from build123d import *

# Parameters (mm, degrees)
SKETCH1_W           = 254
SKETCH1_H           = 127
BOSS_EXTRUDE1_DEPTH = 6.35
SKETCH4_W           = 52.216720723
SKETCH4_H           = 76.2
SKETCH4_R           = 8.89
SKETCH4_R_2         = 12.7
SKETCH4_R_3         = 7.62
SKETCH4_R_4         = 3.175
CUT_EXTRUDE3_DEPTH  = 285.051619429


with BuildPart() as part:
    # Sketch1 → Boss-Extrude1 (new body)
    with BuildSketch(Plane.XY):
        with Locations((127, 63.5)):
            Rectangle(SKETCH1_W, SKETCH1_H)
    extrude(amount=BOSS_EXTRUDE1_DEPTH)

    # Sketch4 → Cut-Extrude3 (cut, through all)
    # profile 1 of 8: a face of its own
    with BuildSketch(Plane.XY.offset(6.35)):
        with Locations((69.998360362, 70.4)):
            Rectangle(SKETCH4_W, SKETCH4_H)
        with Locations((69.925, 95.8)):
            Circle(SKETCH4_R, mode=Mode.SUBTRACT)
        with Locations((69.925, 58.97)):
            Circle(SKETCH4_R_2, mode=Mode.SUBTRACT)
    # profile 2 of 8: a face of its own
    with BuildSketch(Plane.XY.offset(6.35)):
        with Locations((69.925, 95.8)):
            Circle(SKETCH4_R)
    # profile 3 of 8: a face of its own
    with BuildSketch(Plane.XY.offset(6.35)):
        with Locations((69.925, 58.97)):
            Circle(SKETCH4_R_2)
        with Locations((69.925, 58.97)):
            Circle(SKETCH4_R_3, mode=Mode.SUBTRACT)
    # profile 4 of 8: a face of its own
    with BuildSketch(Plane.XY.offset(6.35)):
        with Locations((69.925, 58.97)):
            Circle(SKETCH4_R_3)
    # profile 5 of 8: a face of its own
    with BuildSketch(Plane.XY.offset(6.35)):
        with Locations((99.77, 51.35)):
            Circle(SKETCH4_R_4)
    # profile 6 of 8: a face of its own
    with BuildSketch(Plane.XY.offset(6.35)):
        with Locations((40.08, 51.35)):
            Circle(SKETCH4_R_4)
    # profile 7 of 8: a face of its own
    with BuildSketch(Plane.XY.offset(6.35)):
        with Locations((99.77, 114.85)):
            Circle(SKETCH4_R_4)
    # profile 8 of 8: a face of its own
    with BuildSketch(Plane.XY.offset(6.35)):
        with Locations((40.08, 114.85)):
            Circle(SKETCH4_R_4)
    extrude(amount=-CUT_EXTRUDE3_DEPTH, mode=Mode.SUBTRACT)


solid = part.part
Model file for the job. Use its own axes, mm. A direction names the side the tool comes from. Give positions to 0.01 mm unless a question says otherwise; leave off trailing zeros. Loops run counter-clockwise (first coordinate to the right, second up) from the corner with the lowest first, then second, coordinate; pieces in that order, holes last.
1) Saw through at D-D (z = 1). Write the cut outline in (x, y) (3 decimals), plus the area to 3 significant figures.
2) Flat gauge pin, fed straight in: pin 1 Ø7.5 at (x, y) = (99.77, 114.85) entering from +Z. Where does the tip first touch, or does it go through?
3) Pull direction X, two halves, no side cores. Call faces 1 (the flat face through (125, 0, 3)), 2 (the flat face through (70, 32.3, 3)), 3 (the flat face through (0, 63, 3)): +X half, -X half, draft (parallel to the pull), parting line (faces both ways), or undercut.
4) Wall check: line 1 (Y direction, x = 99.77, z = 3.5) (3 decimals); line 2 (Y direction, x = 63.5, z = 5.5); line 3 (X direction, y = 50.5, z = 3.5). Give the ranges that are in metal, low to high.
5) Saw through at C-C (y = 114.85). Write the cut outline in (x, z) (3 decimals), plus the area to 3 significant figures.
6) Saw through at B-B (x = 40.08). Write the cut outline in (y, z) (3 decimals).
7) Saw through at A-A (y = 51.35). Write the cut outline in (x, z) (3 decimals).
8) Tool access for faces 4 (the flat face through (254, 63, 3)), 5 (the flat face through (70, 108.5, 3)): list every direction of +Z, -Z, +X, -X, +Y, -Y with a clear straight run to the whole face (end or side of a thin tool).
Answer block:
1. outline: (0, 0) - (254, 0) - (254, 127) - (0, 127) - close; hole circle Ø6.35 at (40.08, 51.35); hole circle Ø6.35 at (40.08, 114.85); hole (43.89, 32.3) - (96.107, 32.3) - (96.107, 108.5) - (43.89, 108.5) - close; hole circle Ø6.35 at (99.77, 51.35); hole circle Ø6.35 at (99.77, 114.85)
1. area: 28,200 mm2
2. pin 1: stops at z = 6.35
3. face 1: draft
3. face 2: undercut
3. face 3: -X half
4. line 1: y = 0 to 48.175, 54.525 to 111.675, 118.025 to 127
4. line 2: y = 0 to 32.3, 108.5 to 127
4. line 3: x = 0 to 37.02, 43.14 to 43.89, 96.11 to 96.71, 102.83 to 254
5. outline: (0, 0) - (36.905, 0) - (36.905, 6.35) - (0, 6.35) - close; (43.255, 0) - (96.595, 0) - (96.595, 6.35) - (43.255, 6.35) - close; (102.945, 0) - (254, 0) - (254, 6.35) - (102.945, 6.35) - close
5. area: 1,530 mm2
6. outline: (0, 0) - (48.175, 0) - (48.175, 6.35) - (0, 6.35) - close; (54.525, 0) - (111.675, 0) - (111.675, 6.35) - (54.525, 6.35) - close; (118.025, 0) - (127, 0) - (127, 6.35) - (118.025, 6.35) - close
7. outline: (0, 0) - (36.905, 0) - (36.905, 6.35) - (0, 6.35) - close; (43.255, 0) - (43.89, 0) - (43.89, 6.35) - (43.255, 6.35) - close; (96.107, 0) - (96.595, 0) - (96.595, 6.35) - (96.107, 6.35) - close; (102.945, 0) - (254, 0) - (254, 6.35) - (102.945, 6.35) - close
8. face 4: +Z, -Z, +X, +Y, -Y
8. face 5: +Z, -Z
